from build123d import *

# Parameters (mm, degrees)
SKETCH_2_R                   = 44.45
SKETCH_2_R_2                 = 127
EXTRUDE_1_DEPTH              = 76.2
SKETCH_4_W                   = 660.4
SKETCH_4_H                   = 76.2
EXTRUDE_2_DEPTH              = 850.9
FILLET_2_R                   = 101.6
SKETCH_5_R                   = 44.45
SKETCH_5_R_2                 = 101.6
CUT_EXTRUDE_1_DEPTH          = 850.9
SCALE_1_SCALE                = 0.039370079
HOLE_WIZARD_M6_3_D           = 3.5
HOLE_WIZARD_M6_3_DEPTH       = 16.51
HOLE_WIZARD_M6_3_CSINK_D     = 6.3
HOLE_WIZARD_M6_3_CSINK_ANGLE = 90
HOLE_WIZARD_M6_3_TIP         = 1.051506083


with BuildPart() as part:
    # 草图2 → 凸台-拉伸1 (new body)
    with BuildSketch(Plane(origin=(0, 0, 0), x_dir=(1, 0, 0), z_dir=(0, 1, 0))):
        with BuildLine():
            Line((-330.2, 368.3), (-330.2, -342.9))
            Line((-330.2, -342.9), (330.2, -342.9))
            Line((330.2, -342.9), (330.2, 368.3))
            ThreePointArc((330.2, 368.3), (315.321024484, 404.221024484), (279.4, 419.1))
            Line((279.4, 419.1), (-279.4, 419.1))
            ThreePointArc((-279.4, 419.1), (-315.321024484, 404.221024484), (-330.2, 368.3))
        make_face()
        with Locations(Location((-209.55, -177.8, 0), (0, 0, 90))):
            Circle(SKETCH_2_R, mode=Mode.SUBTRACT)
        with Locations(Location((0, 0, 0), (0, 0, 90))):
            Circle(SKETCH_2_R_2, mode=Mode.SUBTRACT)
        with Locations(Location((209.55, -177.8, 0), (0, 0, 90))):
            Circle(SKETCH_2_R, mode=Mode.SUBTRACT)
        with Locations(Location((-209.55, 177.8, 0), (0, 0, 90))):
            Circle(SKETCH_2_R, mode=Mode.SUBTRACT)
        with Locations(Location((209.55, 177.8, 0), (0, 0, 90))):
            Circle(SKETCH_2_R, mode=Mode.SUBTRACT)
    extrude(amount=EXTRUDE_1_DEPTH)

    # 草图4 → 凸台-拉伸2 (add)
    with BuildSketch(Plane(origin=(0, 0, 0), x_dir=(1, 0, 0), z_dir=(0, 1, 0))):
        with Locations((0, -381)):
            Rectangle(SKETCH_4_W, SKETCH_4_H)
    extrude(amount=EXTRUDE_2_DEPTH)

    # 圆角2
    fillet_2_edges = [part.edges().sort_by_distance(p)[0] for p in [
        (0, 0, 419.1),
    ]]
    fillet(fillet_2_edges, radius=FILLET_2_R)

    # 草图5 → 切除-拉伸1 (cut)
    with BuildSketch(Plane.XY.offset(419.1)):
        with BuildLine():
            ThreePointArc((-330.2, 520.7), (-233.486660985, 754.186657311), (-5.196e-06, 850.9))
            Line((-5.196e-06, 850.9), (-330.2, 850.9))
            Line((-330.2, 850.9), (-330.2, 520.7))
        make_face()
        with BuildLine():
            Line((330.2, 520.7), (330.2, 850.9))
            Line((330.2, 850.9), (-5.196e-06, 850.9))
            ThreePointArc((-5.196e-06, 850.9), (233.486657311, 754.186660985), (330.2, 520.7))
        make_face()
        with Locations((215.9, 520.7)):
            Circle(SKETCH_5_R)
        with Locations((-215.9, 520.7)):
            Circle(SKETCH_5_R)
        with Locations((0, 520.7)):
            Circle(SKETCH_5_R_2)
    extrude(amount=-CUT_EXTRUDE_1_DEPTH, mode=Mode.SUBTRACT)


with BuildPart() as part_1:
    # 缩放比例1: scaled about (0, 222.368151505, 174.146040327)
    add(part.part.scale(SCALE_1_SCALE).moved(Location((0, 213.613499871, 167.289897007))))

    # M6 内六角花形半沉头螺钉的锥形沉头孔3
    with Locations(Plane.XY.offset(183.789897007)):
        with Locations((-8.5, 234.113499871), (8.5, 234.113499871)):
            CounterSinkHole(HOLE_WIZARD_M6_3_D / 2, HOLE_WIZARD_M6_3_CSINK_D / 2, depth=HOLE_WIZARD_M6_3_DEPTH, counter_sink_angle=HOLE_WIZARD_M6_3_CSINK_ANGLE)
            with Locations((0, 0, -(HOLE_WIZARD_M6_3_DEPTH + HOLE_WIZARD_M6_3_TIP / 2))):  # 118° drill point
                Cone(0, HOLE_WIZARD_M6_3_D / 2, HOLE_WIZARD_M6_3_TIP, mode=Mode.SUBTRACT)


solid = part_1.part
Can you work these out from the model? Positions are in its coordinate system, mm. A direction names the side the tool comes from. Coordinates: 2 decimals unless noted, no trailing zeros. Order: outer loops, then holes, each group sorted by start corner. A loop starts at its lowest first (then second) coordinate and runs counter-clockwise, first axis right, second up. Notation, with made-up numbers: (17.5, 28.25) - (31.5, 28.25) arc R9 ccw to (31.5, 45.25) - close; hole circle Ø4 at (76, -5.75). An arc over 180 degrees is marked (long way). Answer as a JSON object with one key per item and string values. Group by question number.
Q1. Imagine slicing it at C-C (y = 227.5). Please give me the cut outline in (x, z), and give its area (3 significant figures).
Q2. On a 3-axis mill with a long thin cutter (end or side, diameter ignored), from which of +Z, -Z, +X, -X, +Y, -Y can I reach the whole of each face in a straight line? I mean faces 4 (the face through (0, 213.613, 162)), 5 (the face through (0, 228, 180.79)). Say none if no direction works.
Q3. Imagine slicing it at A-A (z = 164). Please give me the cut outline in (x, y).
Q4. Will these pins go through, and if not, where does the flat tip stop? P1, Ø6, axis at x = 1, y = 241.5, coming from the -Z side; P2, Ø9, axis at x = 0, y = 234.11, coming from the +Z side; P3, Ø3, axis at x = -3.5, z = 155, coming from the +Y side.
Q5. We'd pull the mould along Z, two halves only. Please class faces 1 (the face through (0, 216.613, 162)), 2 (the face through (-8.33, 215.09, 162.04)), 3 (the face through (12.43, 215.09, 151.39)): +Z half, -Z half, draft (parallel to the pull), parting line (faces both ways), or undercut.
Q6. Imagine slicing it at B-B (x = 3.25). Please give me the cut outline in (y, z).
Q7. I need wall thicknesses on line 1 (Z direction, x = -8.25, y = 214.85); line 2 (X direction, y = 216.5, z = 175.5); line 3 (Y direction, x = 11.5, z = 176). Which ranges of each line are inside material? Lowest first, please. Write a range as from..to.
Q8. Imagine slicing it at D-D (x = -8.25). Give the number of separate pieces and of enclosed holes in the cut face, and give its area (3 significant figures).
Determined:
{
 "1": {"outline": "(-13, 180.79) - (13, 180.79) - (13, 183.79) - (-13, 183.79) - close", "area": "78.0 mm2"},
 "2": {"face 4": "+Z, -Z, +X, -X, -Y", "face 5": "-Z, +X, -X, +Y"},
 "3": {"outline": "(-13, 213.61) - (-3.77, 213.61) - (-3.77, 216.61) - (-13, 216.61) - close; (3.77, 213.61) - (13, 213.61) - (13, 216.61) - (3.77, 216.61) - close"},
 "4": {"P1": "stops at z = 180.79", "P2": "stops at z = 183.79", "P3": "stops at y = 216.61"},
 "5": {"face 1": "draft", "face 2": "undercut", "face 3": "-Z half"},
 "6": {"outline": "(213.61, 150.79) - (216.61, 150.79) - (216.61, 163.49) - (213.61, 163.49) - close; (213.61, 171.09) - (216.61, 171.09) - (216.61, 180.79) - (231.78, 180.79) - (231.78, 183.79) - (217.61, 183.79) arc R4 ccw to (213.61, 179.79) - close; (236.45, 180.79) - (246.7, 180.79) - (246.7, 183.79) - (236.45, 183.79) - close"},
 "7": {"line 1": "z = 150.79..158.54, 162.04..172.54, 176.04..182.68", "line 2": "x = -13..-9.51, -6.99..6.99, 9.51..13", "line 3": "y = 213.61..216.61"},
 "8": {"separate pieces": "4", "enclosed holes": "0", "area": "145 mm2"}
}
